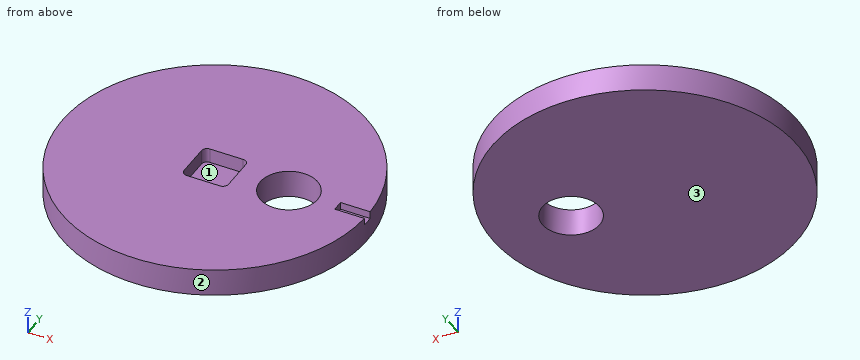
```python
from build123d import *

# Parameters (mm, degrees)
SKETCH004_R             = 41.2
SKETCH004_R_2           = 7.75
PAD002_DEPTH            = 7.5
POCKET007_DEPTH         = 2
POCKET008_DEPTH         = 4
BODY002_PLACEMENT_ANGLE = 90


with BuildPart() as part:
    # Sketch004 → Pad002 (new body)
    with BuildSketch(Plane.XY):
        Circle(SKETCH004_R)
        with Locations((0, -20)):
            Circle(SKETCH004_R_2, mode=Mode.SUBTRACT)
    extrude(amount=PAD002_DEPTH)

    # Sketch018 (on Face4 of Pad002) → Pocket007 (cut)
    with BuildSketch(Plane.XY.offset(7.5)):
        with BuildLine():
            Line((-1.5, -33.172685), (-1.5, -41.172685))
            ThreePointArc((-1.5, -41.172685), (0, -41.2), (1.5, -41.172685))
            Line((1.5, -41.172685), (1.5, -33.172685))
            Line((1.5, -33.172685), (-1.5, -33.172685))
        make_face()
    extrude(amount=-POCKET007_DEPTH, mode=Mode.SUBTRACT)

    # Sketch019 (on Face3 of Pocket007) → Pocket008 (cut)
    with BuildSketch(Plane.XY.offset(7.5)):
        with BuildLine():
            Line((-6, 4.5), (-6, -4.5))
            ThreePointArc((-6, -4.5), (-5.56066, -5.56066), (-4.5, -6))
            Line((-4.5, -6), (4.5, -6))
            ThreePointArc((4.5, -6), (5.56066, -5.56066), (6, -4.5))
            Line((6, -4.5), (6, 4.5))
            ThreePointArc((6, 4.5), (5.56066, 5.56066), (4.5, 6))
            Line((4.5, 6), (-4.5, 6))
            ThreePointArc((-4.5, 6), (-5.56066, 5.56066), (-6, 4.5))
        make_face()
    extrude(amount=-POCKET008_DEPTH, mode=Mode.SUBTRACT)


with BuildPart() as part_1:
    # Body002 placement: moved
    add(part.part.moved(Location((0, 0, -3))).rotate(Axis((0, 0, -3), (0, 0, 1)), BODY002_PLACEMENT_ANGLE))


solid = part_1.part
```
Work out the finished part from the listing and answer in its coordinate system (mm). Face numbers are marked on the shaded views. Coordinates: 2 decimals unless noted, no trailing zeros. Order: outer loops, then holes, each group sorted by start corner. A loop starts at its lowest first (then second) coordinate and runs counter-clockwise, first axis right, second up. Notation, with made-up numbers: M 0,47 L 42,47 A7 cw 42,56 Z; hole C 45.25,54 d2. An arc over 180 degrees is marked long. Use CSV: the item, a comma, the result in double quotes.
1) Determine the mould class of the marked faces 1, 2 and 3 for opening direction X: released by +X, released by -X, zero draft, split by the parting line, or undercut.
Worked out:
face 1,"undercut"
face 2,"split by the parting line"
face 3,"zero draft"
2) Section C-C on x = 20 is taken. Write down the section's boundary in (y, z).
Worked out:
outline,"M -36.02,-3 L -7.75,-3 L -7.75,4.5 L -36.02,4.5 Z; M 7.75,-3 L 36.02,-3 L 36.02,4.5 L 7.75,4.5 Z"
3) Section A-A on y = 0 is taken. Write down the section's boundary in (x, z).
Worked out:
outline,"M -41.2,-3 L 12.25,-3 L 12.25,4.5 L 6,4.5 L 6,0.5 L -6,0.5 L -6,4.5 L -41.2,4.5 Z; M 27.75,-3 L 41.2,-3 L 41.2,2.5 L 33.17,2.5 L 33.17,4.5 L 27.75,4.5 Z"
4) Consider line 1 (X direction, y = 0, z = 0.25); line 2 (Y direction, x = 20, z = -0.5); line 3 (X direction, y = -6, z = -0.5). Determine where each line is inside the solid, lowest interval first. Write a range as [from, to].
Worked out:
line 1,"x = [-41.2, 12.25], [27.75, 41.2]"
line 2,"y = [-36.02, -7.75], [7.75, 36.02]"
line 3,"x = [-40.76, 15.09], [24.91, 40.76]"
5) Section D-D on x = 0 is taken. Write down the section's boundary in (y, z), plus the area to 3 significant figures.
Worked out:
outline,"M -41.2,-3 L 41.2,-3 L 41.2,4.5 L 6,4.5 L 6,0.5 L -6,0.5 L -6,4.5 L -41.2,4.5 Z"
area,"570 mm^2"
6) Flat-ended cylindrical pins translate along their axes: pin 1 Ø3 at (x, z) = (2, 2) entering from +Y; pin 2 Ø1 at (x, z) = (36, 3) entering from +Y; pin 3 Ø18 at (x, y) = (20, 0) entering from -Z; pin 4 Ø4 at (y, z) = (-31.5, -0.5) entering from -X. Find the tip coordinate at first contact, or state that the pin passes through.
Worked out:
pin 1,"stops at y = 41.2"
pin 2,"stops at y = 20.91"
pin 3,"stops at z = -3"
pin 4,"stops at x = -28.76"
7) Section B-B on z = 3.5 is taken. Write down the section's boundary in (x, y), plus the area to 3 significant figures.
Worked out:
outline,"M 33.17,-1.5 L 33.17,1.5 L 41.17,1.5 A41.2 ccw long 41.17,-1.5 Z; hole M -6,-4.5 A1.5 ccw -4.5,-6 L 4.5,-6 A1.5 ccw 6,-4.5 L 6,4.5 A1.5 ccw 4.5,6 L -4.5,6 A1.5 ccw -6,4.5 Z; hole C 20,0 d15.5"
area,"4,980 mm^2"
